The model under review builds one solid part; all positions refer to its coordinate system, in mm. A direction names the side the tool comes from. Round coordinates to 2 decimals unless told otherwise and drop trailing zeros. Write each loop counter-clockwise with the first axis right and the second up, starting at its lowest first coordinate (ties: lowest second). Pieces come first, ordered by that corner, then holes. Notation, with made-up numbers: M 54.5,54 L 66.5,54 A21 ccw 66.5,72 Z; hole C -37,-14.5 d9. An arc over 180 degrees is marked long. Write item = value, one per line. Start each with the question number.
Item 1: Tool access review of faces 1 (the flat face through (-17.943, -2, 19)), 2 (the cylindrical face through (13.024, 12.07, 5.283)), 3 (the flat face through (-6.958, -7.462, 19.227)): name each direction out of +Z, -Z, +X, -X, +Y, -Y from which nothing blocks a thin tool from reaching the whole face with its end or side.
Item 2: Take a section at D-D, the plane z = 5.5. Give the boundary of the cut face in (x, y), plus the area to 3 significant figures.
Item 3: To check wall thickness, follow line 1 along X through (y, z) = (12, 33.5); line 2 along X through (y, z) = (0, 9); line 3 along X through (y, z) = (13.5, 5). State the ranges of each line that lie inside material, in increasing order.
Item 4: Take a section at C-C, the plane y = 8.25. Give the boundary of the cut face in (x, z).
Item 5: For pin 1 Ø5.5 at (y, z) = (-2, 27.5) entering from -X; pin 2 Ø4 at (y, z) = (-7, 7) entering from +X; pin 3 Ø1.6 at (x, z) = (-14, 5.5) entering from +Y; pin 4 Ø11 at (x, y) = (0, 0) entering from +Z, all flat-tipped, find the tip position at first contact; note any pin that passes through.
Item 6: The part is to be moulded in two halves that separate along Y. For faces 4 (the flat face through (-0.3, 6.5, 0)), 5 (the flat face through (-14, 7, 33)), 6 (the flat face through (19, 8, 19)), 7 (the cylindrical face through (0, 6, 19)), say which applies: +Y half, -Y half, draft (parallel to the pull), parting line (faces both ways), or undercut.
Item 7: Take a section at A-A, the plane y = 0. Give the boundary of the cut face in (x, z), plus the area to 3 significant figures.
Item 8: Take a section at B-B, the plane x = 14. Give the boundary of the cut face in (y, z).
from build123d import *

# Parameters (mm, degrees)
BOSS_EXTRUDE1_DEPTH = 39
SKETCH2_R           = 1
CUT_EXTRUDE1_DEPTH  = 10


with BuildPart() as part:
    # Sketch1 → Boss-Extrude1 (new body)
    with BuildSketch(Plane.XY):
        with BuildLine():
            Line((20, 17), (-20, 17))
            Line((-20, 17), (-20, 9))
            Line((-20, 9), (-17.943455856, 6.943455856))
            Line((-17.943455856, 6.943455856), (-17.943455856, -10.6))
            Line((-17.943455856, -10.6), (-9.590643782, -10.6))
            Line((-9.590643782, -10.6), (-4.25, -4.235268587))
            ThreePointArc((-4.25, -4.235268587), (0, 6), (4.25, -4.235268587))
            Line((4.25, -4.235268587), (9.590643782, -10.6))
            Line((9.590643782, -10.6), (17.943455856, -10.6))
            Line((17.943455856, -10.6), (17.943455856, 6.943455856))
            Line((17.943455856, 6.943455856), (20, 9))
            Line((20, 9), (20, 17))
        make_face()
    extrude(amount=BOSS_EXTRUDE1_DEPTH)

    # Sketch2 → Cut-Extrude1 (cut)
    with BuildSketch(Plane(origin=(0, 17, 0), x_dir=(1, 0, 0), z_dir=(0, 1, 0))):
        with Locations(Location((-14, -33.5, 0), (0, 0, 270))):
            Circle(SKETCH2_R)
        with Locations(Location((14, -33.5, 0), (0, 0, 270))):
            Circle(SKETCH2_R)
        with Locations(Location((-14, -5.5, 0), (0, 0, 270))):
            Circle(SKETCH2_R)
        with Locations(Location((14, -5.5, 0), (0, 0, 270))):
            Circle(SKETCH2_R)
    extrude(amount=-CUT_EXTRUDE1_DEPTH, mode=Mode.SUBTRACT)


solid = part.part
Response values:
q1.face_1 = +Z, -Z, -X, -Y
q1.face_2 = +Y
q1.face_3 = +Z, -Z, -Y
q2.outline = M -20,9 L -17.94,6.94 L -17.94,-10.6 L -9.59,-10.6 L -4.25,-4.24 A6 cw long 4.25,-4.24 L 9.59,-10.6 L 17.94,-10.6 L 17.94,6.94 L 20,9 L 20,17 L 15,17 L 15,7 L 13,7 L 13,17 L -13,17 L -13,7 L -15,7 L -15,17 L -20,17 Z
q2.area = 797 mm2
q3.line_1 = -20 to -15, -13 to 13, 15 to 20
q3.line_2 = -17.94 to -6, 6 to 17.94
q3.line_3 = -20 to -14.87, -13.13 to 13.13, 14.87 to 20
q4.outline = M -19.25,0 L 19.25,0 L 19.25,39 L -19.25,39 Z; hole C -14,5.5 d2; hole C -14,33.5 d2; hole C 14,5.5 d2; hole C 14,33.5 d2
q5.pin_1 = -17.94
q5.pin_2 = 17.94
q5.pin_3 = 7
q5.pin_4 = through
q6.face_4 = draft
q6.face_5 = +Y half
q6.face_6 = -Y half
q6.face_7 = undercut
q7.outline = M -17.94,0 L -6,0 L -6,39 L -17.94,39 Z; M 6,0 L 17.94,0 L 17.94,39 L 6,39 Z
q7.area = 932 mm2
q8.outline = M -10.6,0 L 17,0 L 17,4.5 L 7,4.5 L 7,6.5 L 17,6.5 L 17,32.5 L 7,32.5 L 7,34.5 L 17,34.5 L 17,39 L -10.6,39 Z
